Could you check a few things on this model? Use its own coordinates, in mm. A direction names the side the tool comes from. Give positions to 0.01 mm unless a question says otherwise; leave off trailing zeros. Write each loop counter-clockwise with the first axis right and the second up, starting at its lowest first coordinate (ties: lowest second). Pieces come first, ordered by that corner, then holes. Notation, with made-up numbers: (34, -2.5) - (91, -2.5) arc R26 ccw to (91, 27.5) - close; hole circle Ø7 at (-39.5, -25.5). An arc over 180 degrees is marked (long way). Write item = value, one per line.
from build123d import *

# Parameters (mm, degrees)
SKETCH1_R           = 3
BOSS_EXTRUDE1_DEPTH = 110
BOSS_EXTRUDE2_START = 5
SKETCH2_R           = 4.5
SKETCH2_R_2         = 3
BOSS_EXTRUDE2_DEPTH = 5
FILLET1_R           = 1
BOSS_EXTRUDE3_START = -5
SKETCH3_R           = 3.5
SKETCH3_R_2         = 3
BOSS_EXTRUDE3_DEPTH = 5
CUT_EXTRUDE1_START  = -95
CUT_EXTRUDE1_DEPTH  = 95
FILLET2_R           = 1


with BuildPart() as part:
    # Sketch1 → Boss-Extrude1 (new body)
    with BuildSketch(Plane(origin=(0, 0, 0), x_dir=(1, 0, 0), z_dir=(0, 1, 0))):
        with Locations(Location((0, 0, 0), (0, 0, 270))):
            Circle(SKETCH1_R)
    extrude(amount=BOSS_EXTRUDE1_DEPTH)

    # Sketch2 → Boss-Extrude2 (add)
    # profile 1 of 2: a face of its own
    with BuildSketch(Plane.XZ.offset(BOSS_EXTRUDE2_START)):
        with Locations(Location((0, 0, 0), (0, 0, 270))):
            Circle(SKETCH2_R)
        with Locations(Location((0, 0, 0), (0, 0, 90))):
            Circle(SKETCH2_R_2, mode=Mode.SUBTRACT)
    # profile 2 of 2: a face of its own
    with BuildSketch(Plane.XZ.offset(BOSS_EXTRUDE2_START)):
        with Locations(Location((0, 0, 0), (0, 0, 90))):
            Circle(SKETCH2_R_2)
    extrude(amount=-BOSS_EXTRUDE2_DEPTH)

    # Fillet1
    fillet1_edges = [part.edges().sort_by_distance(p)[0] for p in [
        (0, 0, 4.5),
        (0, -5, 4.5),
    ]]
    fillet(fillet1_edges, radius=FILLET1_R)

    # Sketch3 → Boss-Extrude3 (add)
    with BuildSketch(Plane(origin=(0, 110, 0), x_dir=(1, 0, 0), z_dir=(0, 1, 0)).offset(BOSS_EXTRUDE3_START)):
        with Locations(Location((0, 0, 0), (0, 0, 270))):
            Circle(SKETCH3_R)
        with Locations(Location((0, 0, 0), (0, 0, 270))):
            Circle(SKETCH3_R_2, mode=Mode.SUBTRACT)
    extrude(amount=BOSS_EXTRUDE3_DEPTH)

    # Sketch4 → Cut-Extrude1 (cut)
    with BuildSketch(Plane(origin=(0, 110, 0), x_dir=(1, 0, 0), z_dir=(0, 1, 0)).offset(CUT_EXTRUDE1_START)):
        with BuildLine():
            Line((-1.3, 3.249615362), (-1.3, -3.249615362))
            ThreePointArc((-1.3, -3.249615362), (0, -3.5), (1.3, -3.249615362))
            Line((1.3, -3.249615362), (1.3, 3.249615362))
            ThreePointArc((1.3, 3.249615362), (0, 3.5), (-1.3, 3.249615362))
        make_face()
    extrude(amount=CUT_EXTRUDE1_DEPTH, mode=Mode.SUBTRACT)

    # Fillet2
    fillet2_edges = [part.edges().sort_by_distance(p)[0] for p in [
        (3.5, 110, 0),
        (-3.5, 110, 0),
        (-1.3, 110, 0),
        (1.3, 110, 0),
    ]]
    fillet(fillet2_edges, radius=FILLET2_R)


solid = part.part
1. For pin 1 (3 mm diameter, centred on y = 22.5, z = -3.5, fed in from -X); pin 2 (5 mm diameter, centred on x = -3.5, y = 58, fed in from -Z); pin 3 (1.3 mm diameter, centred on x = 0, z = 1, fed in from +Y); pin 4 (4 mm diameter, centred on x = 3.5, z = 2, fed in from -Y), each with a flat end and sliding along its axis, tell me the tip position at first contact or that it passes through.
Filled sheet:
pin_1 = -2.24
pin_2 = -2.7
pin_3 = 15
pin_4 = -5
2. If we section it at A-A, the plane x = 0: Please give me the cut outline in (y, z).
Filled sheet:
outline = (-5, -3.5) arc R1 ccw to (-4, -4.5) - (-1, -4.5) arc R1 ccw to (0, -3.5) - (0, -3) - (15, -3) - (15, 3) - (0, 3) - (0, 3.5) arc R1 ccw to (-1, 4.5) - (-4, 4.5) arc R1 ccw to (-5, 3.5) - close
3. If we section it at B-B, the plane z = 0: Please give me the cut outline in (x, y).
Filled sheet:
outline = (-4.5, -4) arc R1 ccw to (-3.5, -5) - (3.5, -5) arc R1 ccw to (4.5, -4) - (4.5, -1) arc R1 ccw to (3.5, 0) - (3, 0) - (3, 105) - (3.5, 105) - (3.5, 109) arc R1 ccw to (2.5, 110) - (2.3, 110) arc R1 ccw to (1.3, 109) - (1.3, 15) - (-1.3, 15) - (-1.3, 109) arc R1 ccw to (-2.3, 110) - (-2.5, 110) arc R1 ccw to (-3.5, 109) - (-3.5, 105) - (-3, 105) - (-3, 0) - (-3.5, 0) arc R1 ccw to (-4.5, -1) - close
4. Thinking about a two-plate mould opening in Y: for faces 4 (the face through (-1.8, 51.8, -2.4)), 5 (the face through (1.3, 61, 0)), 6 (the face through (0, -5, 0)), which applies, pulls with the +Y half, pulls with the -Y half, needs draft (parallel to the pull), parting line crosses it, or undercut?
Filled sheet:
face_4 = undercut
face_5 = needs draft
face_6 = pulls with the -Y half
5. I need wall thicknesses on line 1 (X direction, y = 104, z = 1.25); line 2 (Y direction, x = 0.25, z = 0.25); line 3 (X direction, y = 53, z = 0.5). Which ranges of each line are inside material? Lowest first, please.
Filled sheet:
line_1 = -2.73 to -1.3, 1.3 to 2.73
line_2 = -5 to 15
line_3 = -2.96 to -1.3, 1.3 to 2.96
6. Which directions (+Z, -Z, +X, -X, +Y, -Y) give clear straight access to the entire face, cutting with the end or side of a thin tool? Please do faces 1 (the face through (1, 0, -3)), 2 (the face through (-3.2, 105, 0)), 3 (the face through (-3.5, 107, -0.1)).
Filled sheet:
face_1 = none
face_2 = -X
face_3 = -X, +Y
7. If we section it at C-C, the plane y = 37: Please give me the cut outline in (x, z), and give its area (3 significant figures).
Filled sheet:
outline = (-1.3, -2.7) - (-1.3, 2.7) arc R3 ccw to start; (1.3, -2.7) arc R3 ccw to (1.3, 2.7) - close
area = 13.2 mm2
8. If we section it at D-D, the plane y = 8.5: Please give me the cut outline in (x, z), and give its area (3 significant figures).
Filled sheet:
outline = circle Ø6 at (0, 0)
area = 28.3 mm2
